Geometry: final body of the model. Coordinates: model frame, mm. Round coordinates to 2 decimals unless told otherwise and drop trailing zeros. Loops run counter-clockwise (first coordinate to the right, second up) from the corner with the lowest first, then second, coordinate; pieces in that order, holes last. Notation, with made-up numbers: (-36.75, 87) - (16.25, 87) arc R16 cw to (16.25, 93) - close; hole circle Ø11 at (87.5, -4). An arc over 180 degrees is marked (long way). Write item = value, one per line. Start each with the question number.
Item 1: Section B-B (y = 0.65). Count the separate pieces of the cut face and the enclosed holes in it, plus the area to 3 significant figures.
Item 2: First-contact query: pin 1 (8 mm diameter, centred on x = 13.5, z = 1.98, fed in from -Y); pin 2 (5.5 mm diameter, centred on x = -40.5, z = 1.98, fed in from +Y). Flat tips, straight axial feed; report the tip coordinate or a pass-through.
Item 3: Section A-A (x = -4.5). Return loops of the section in (y, z), plus the area to 3 significant figures.
Item 4: Draft query along X for faces 1 (the flat face through (-1, 0.794, -3)), 2 (the cylindrical face through (26.011, 0.391, -30.805)). Return one class per face: pulls with the +X half, pulls with the -X half, needs draft (parallel to the pull), parting line crosses it, or undercut.
from build123d import *

# Parameters (mm, degrees)
SKETCH1_W           = 108
SKETCH1_H           = 82
SKETCH1_R           = 1.625
SKETCH1_R_2         = 3.15
BOSS_EXTRUDE1_DEPTH = 0.79375


with BuildPart() as part:
    # Sketch1 → Boss-Extrude1 (new body)
    with BuildSketch(Plane(origin=(0, 0, 0), x_dir=(1, 0, 0), z_dir=(0, 1, 0))):
        with Locations((0, 2.515945223)):
            Rectangle(SKETCH1_W, SKETCH1_H)
        with Locations(Location((-45, 29.515945223, 0), (0, 0, 270))):
            Circle(SKETCH1_R, mode=Mode.SUBTRACT)
        with Locations(Location((-49.5, 25.015945223, 0), (0, 0, 270))):
            Circle(SKETCH1_R_2, mode=Mode.SUBTRACT)
        with Locations(Location((-27, 29.515945223, 0), (0, 0, 270))):
            Circle(SKETCH1_R, mode=Mode.SUBTRACT)
        with Locations(Location((-9, 29.515945223, 0), (0, 0, 270))):
            Circle(SKETCH1_R, mode=Mode.SUBTRACT)
        with Locations(Location((9, 29.515945223, 0), (0, 0, 270))):
            Circle(SKETCH1_R, mode=Mode.SUBTRACT)
        with Locations(Location((27, 29.515945223, 0), (0, 0, 270))):
            Circle(SKETCH1_R, mode=Mode.SUBTRACT)
        with Locations(Location((45, 29.515945223, 0), (0, 0, 270))):
            Circle(SKETCH1_R, mode=Mode.SUBTRACT)
        with Locations(Location((-27, 11.515945223, 0), (0, 0, 270))):
            Circle(SKETCH1_R, mode=Mode.SUBTRACT)
        with Locations(Location((-9, 11.515945223, 0), (0, 0, 270))):
            Circle(SKETCH1_R, mode=Mode.SUBTRACT)
        with Locations(Location((9, 11.515945223, 0), (0, 0, 270))):
            Circle(SKETCH1_R, mode=Mode.SUBTRACT)
        with Locations(Location((27, 11.515945223, 0), (0, 0, 270))):
            Circle(SKETCH1_R, mode=Mode.SUBTRACT)
        with Locations(Location((45, 11.515945223, 0), (0, 0, 270))):
            Circle(SKETCH1_R, mode=Mode.SUBTRACT)
        with Locations(Location((-27, -6.484054777, 0), (0, 0, 270))):
            Circle(SKETCH1_R, mode=Mode.SUBTRACT)
        with Locations(Location((-9, -6.484054777, 0), (0, 0, 270))):
            Circle(SKETCH1_R, mode=Mode.SUBTRACT)
        with Locations(Location((9, -6.484054777, 0), (0, 0, 270))):
            Circle(SKETCH1_R, mode=Mode.SUBTRACT)
        with Locations(Location((27, -6.484054777, 0), (0, 0, 270))):
            Circle(SKETCH1_R, mode=Mode.SUBTRACT)
        with Locations(Location((45, -6.484054777, 0), (0, 0, 270))):
            Circle(SKETCH1_R, mode=Mode.SUBTRACT)
        with Locations(Location((-27, -24.484054777, 0), (0, 0, 270))):
            Circle(SKETCH1_R, mode=Mode.SUBTRACT)
        with Locations(Location((-9, -24.484054777, 0), (0, 0, 270))):
            Circle(SKETCH1_R, mode=Mode.SUBTRACT)
        with Locations(Location((9, -24.484054777, 0), (0, 0, 270))):
            Circle(SKETCH1_R, mode=Mode.SUBTRACT)
        with Locations(Location((27, -24.484054777, 0), (0, 0, 270))):
            Circle(SKETCH1_R, mode=Mode.SUBTRACT)
        with Locations(Location((45, -24.484054777, 0), (0, 0, 270))):
            Circle(SKETCH1_R, mode=Mode.SUBTRACT)
        with Locations(Location((-45, 11.515945223, 0), (0, 0, 270))):
            Circle(SKETCH1_R, mode=Mode.SUBTRACT)
        with Locations(Location((-45, -6.484054777, 0), (0, 0, 270))):
            Circle(SKETCH1_R, mode=Mode.SUBTRACT)
        with Locations(Location((-45, -24.484054777, 0), (0, 0, 270))):
            Circle(SKETCH1_R, mode=Mode.SUBTRACT)
        with Locations(Location((-40.5, 25.015945223, 0), (0, 0, 270))):
            Circle(SKETCH1_R_2, mode=Mode.SUBTRACT)
        with Locations(Location((-31.5, 25.015945223, 0), (0, 0, 270))):
            Circle(SKETCH1_R_2, mode=Mode.SUBTRACT)
        with Locations(Location((-22.5, 25.015945223, 0), (0, 0, 270))):
            Circle(SKETCH1_R_2, mode=Mode.SUBTRACT)
        with Locations(Location((-13.5, 25.015945223, 0), (0, 0, 270))):
            Circle(SKETCH1_R_2, mode=Mode.SUBTRACT)
        with Locations(Location((-4.5, 25.015945223, 0), (0, 0, 270))):
            Circle(SKETCH1_R_2, mode=Mode.SUBTRACT)
        with Locations(Location((4.5, 25.015945223, 0), (0, 0, 270))):
            Circle(SKETCH1_R_2, mode=Mode.SUBTRACT)
        with Locations(Location((13.5, 25.015945223, 0), (0, 0, 270))):
            Circle(SKETCH1_R_2, mode=Mode.SUBTRACT)
        with Locations(Location((22.5, 25.015945223, 0), (0, 0, 270))):
            Circle(SKETCH1_R_2, mode=Mode.SUBTRACT)
        with Locations(Location((31.5, 25.015945223, 0), (0, 0, 270))):
            Circle(SKETCH1_R_2, mode=Mode.SUBTRACT)
        with Locations(Location((40.5, 25.015945223, 0), (0, 0, 270))):
            Circle(SKETCH1_R_2, mode=Mode.SUBTRACT)
        with Locations(Location((49.5, 25.015945223, 0), (0, 0, 270))):
            Circle(SKETCH1_R_2, mode=Mode.SUBTRACT)
        with Locations(Location((-40.5, 16.015945223, 0), (0, 0, 270))):
            Circle(SKETCH1_R_2, mode=Mode.SUBTRACT)
        with Locations(Location((-31.5, 16.015945223, 0), (0, 0, 270))):
            Circle(SKETCH1_R_2, mode=Mode.SUBTRACT)
        with Locations(Location((-22.5, 16.015945223, 0), (0, 0, 270))):
            Circle(SKETCH1_R_2, mode=Mode.SUBTRACT)
        with Locations(Location((-13.5, 16.015945223, 0), (0, 0, 270))):
            Circle(SKETCH1_R_2, mode=Mode.SUBTRACT)
        with Locations(Location((-4.5, 16.015945223, 0), (0, 0, 270))):
            Circle(SKETCH1_R_2, mode=Mode.SUBTRACT)
        with Locations(Location((4.5, 16.015945223, 0), (0, 0, 270))):
            Circle(SKETCH1_R_2, mode=Mode.SUBTRACT)
        with Locations(Location((13.5, 16.015945223, 0), (0, 0, 270))):
            Circle(SKETCH1_R_2, mode=Mode.SUBTRACT)
        with Locations(Location((22.5, 16.015945223, 0), (0, 0, 270))):
            Circle(SKETCH1_R_2, mode=Mode.SUBTRACT)
        with Locations(Location((31.5, 16.015945223, 0), (0, 0, 270))):
            Circle(SKETCH1_R_2, mode=Mode.SUBTRACT)
        with Locations(Location((40.5, 16.015945223, 0), (0, 0, 270))):
            Circle(SKETCH1_R_2, mode=Mode.SUBTRACT)
        with Locations(Location((49.5, 16.015945223, 0), (0, 0, 270))):
            Circle(SKETCH1_R_2, mode=Mode.SUBTRACT)
        with Locations(Location((-40.5, 7.015945223, 0), (0, 0, 270))):
            Circle(SKETCH1_R_2, mode=Mode.SUBTRACT)
        with Locations(Location((-31.5, 7.015945223, 0), (0, 0, 270))):
            Circle(SKETCH1_R_2, mode=Mode.SUBTRACT)
        with Locations(Location((-22.5, 7.015945223, 0), (0, 0, 270))):
            Circle(SKETCH1_R_2, mode=Mode.SUBTRACT)
        with Locations(Location((-13.5, 7.015945223, 0), (0, 0, 270))):
            Circle(SKETCH1_R_2, mode=Mode.SUBTRACT)
        with Locations(Location((-4.5, 7.015945223, 0), (0, 0, 270))):
            Circle(SKETCH1_R_2, mode=Mode.SUBTRACT)
        with Locations(Location((4.5, 7.015945223, 0), (0, 0, 270))):
            Circle(SKETCH1_R_2, mode=Mode.SUBTRACT)
        with Locations(Location((13.5, 7.015945223, 0), (0, 0, 270))):
            Circle(SKETCH1_R_2, mode=Mode.SUBTRACT)
        with Locations(Location((22.5, 7.015945223, 0), (0, 0, 270))):
            Circle(SKETCH1_R_2, mode=Mode.SUBTRACT)
        with Locations(Location((31.5, 7.015945223, 0), (0, 0, 270))):
            Circle(SKETCH1_R_2, mode=Mode.SUBTRACT)
        with Locations(Location((40.5, 7.015945223, 0), (0, 0, 270))):
            Circle(SKETCH1_R_2, mode=Mode.SUBTRACT)
        with Locations(Location((49.5, 7.015945223, 0), (0, 0, 270))):
            Circle(SKETCH1_R_2, mode=Mode.SUBTRACT)
        with Locations(Location((-40.5, -1.984054777, 0), (0, 0, 270))):
            Circle(SKETCH1_R_2, mode=Mode.SUBTRACT)
        with Locations(Location((-31.5, -1.984054777, 0), (0, 0, 270))):
            Circle(SKETCH1_R_2, mode=Mode.SUBTRACT)
        with Locations(Location((-22.5, -1.984054777, 0), (0, 0, 270))):
            Circle(SKETCH1_R_2, mode=Mode.SUBTRACT)
        with Locations(Location((-13.5, -1.984054777, 0), (0, 0, 270))):
            Circle(SKETCH1_R_2, mode=Mode.SUBTRACT)
        with Locations(Location((-4.5, -1.984054777, 0), (0, 0, 270))):
            Circle(SKETCH1_R_2, mode=Mode.SUBTRACT)
        with Locations(Location((4.5, -1.984054777, 0), (0, 0, 270))):
            Circle(SKETCH1_R_2, mode=Mode.SUBTRACT)
        with Locations(Location((13.5, -1.984054777, 0), (0, 0, 270))):
            Circle(SKETCH1_R_2, mode=Mode.SUBTRACT)
        with Locations(Location((22.5, -1.984054777, 0), (0, 0, 270))):
            Circle(SKETCH1_R_2, mode=Mode.SUBTRACT)
        with Locations(Location((31.5, -1.984054777, 0), (0, 0, 270))):
            Circle(SKETCH1_R_2, mode=Mode.SUBTRACT)
        with Locations(Location((40.5, -1.984054777, 0), (0, 0, 270))):
            Circle(SKETCH1_R_2, mode=Mode.SUBTRACT)
        with Locations(Location((49.5, -1.984054777, 0), (0, 0, 270))):
            Circle(SKETCH1_R_2, mode=Mode.SUBTRACT)
        with Locations(Location((-40.5, -10.984054777, 0), (0, 0, 270))):
            Circle(SKETCH1_R_2, mode=Mode.SUBTRACT)
        with Locations(Location((-31.5, -10.984054777, 0), (0, 0, 270))):
            Circle(SKETCH1_R_2, mode=Mode.SUBTRACT)
        with Locations(Location((-22.5, -10.984054777, 0), (0, 0, 270))):
            Circle(SKETCH1_R_2, mode=Mode.SUBTRACT)
        with Locations(Location((-13.5, -10.984054777, 0), (0, 0, 270))):
            Circle(SKETCH1_R_2, mode=Mode.SUBTRACT)
        with Locations(Location((-4.5, -10.984054777, 0), (0, 0, 270))):
            Circle(SKETCH1_R_2, mode=Mode.SUBTRACT)
        with Locations(Location((4.5, -10.984054777, 0), (0, 0, 270))):
            Circle(SKETCH1_R_2, mode=Mode.SUBTRACT)
        with Locations(Location((13.5, -10.984054777, 0), (0, 0, 270))):
            Circle(SKETCH1_R_2, mode=Mode.SUBTRACT)
        with Locations(Location((22.5, -10.984054777, 0), (0, 0, 270))):
            Circle(SKETCH1_R_2, mode=Mode.SUBTRACT)
        with Locations(Location((31.5, -10.984054777, 0), (0, 0, 270))):
            Circle(SKETCH1_R_2, mode=Mode.SUBTRACT)
        with Locations(Location((40.5, -10.984054777, 0), (0, 0, 270))):
            Circle(SKETCH1_R_2, mode=Mode.SUBTRACT)
        with Locations(Location((49.5, -10.984054777, 0), (0, 0, 270))):
            Circle(SKETCH1_R_2, mode=Mode.SUBTRACT)
        with Locations(Location((-40.5, -19.984054777, 0), (0, 0, 270))):
            Circle(SKETCH1_R_2, mode=Mode.SUBTRACT)
        with Locations(Location((-31.5, -19.984054777, 0), (0, 0, 270))):
            Circle(SKETCH1_R_2, mode=Mode.SUBTRACT)
        with Locations(Location((-22.5, -19.984054777, 0), (0, 0, 270))):
            Circle(SKETCH1_R_2, mode=Mode.SUBTRACT)
        with Locations(Location((-13.5, -19.984054777, 0), (0, 0, 270))):
            Circle(SKETCH1_R_2, mode=Mode.SUBTRACT)
        with Locations(Location((-4.5, -19.984054777, 0), (0, 0, 270))):
            Circle(SKETCH1_R_2, mode=Mode.SUBTRACT)
        with Locations(Location((4.5, -19.984054777, 0), (0, 0, 270))):
            Circle(SKETCH1_R_2, mode=Mode.SUBTRACT)
        with Locations(Location((13.5, -19.984054777, 0), (0, 0, 270))):
            Circle(SKETCH1_R_2, mode=Mode.SUBTRACT)
        with Locations(Location((22.5, -19.984054777, 0), (0, 0, 270))):
            Circle(SKETCH1_R_2, mode=Mode.SUBTRACT)
        with Locations(Location((31.5, -19.984054777, 0), (0, 0, 270))):
            Circle(SKETCH1_R_2, mode=Mode.SUBTRACT)
        with Locations(Location((40.5, -19.984054777, 0), (0, 0, 270))):
            Circle(SKETCH1_R_2, mode=Mode.SUBTRACT)
        with Locations(Location((49.5, -19.984054777, 0), (0, 0, 270))):
            Circle(SKETCH1_R_2, mode=Mode.SUBTRACT)
        with Locations(Location((-49.5, 16.015945223, 0), (0, 0, 270))):
            Circle(SKETCH1_R_2, mode=Mode.SUBTRACT)
        with Locations(Location((-49.5, 7.015945223, 0), (0, 0, 270))):
            Circle(SKETCH1_R_2, mode=Mode.SUBTRACT)
        with Locations(Location((-49.5, -1.984054777, 0), (0, 0, 270))):
            Circle(SKETCH1_R_2, mode=Mode.SUBTRACT)
        with Locations(Location((-49.5, -10.984054777, 0), (0, 0, 270))):
            Circle(SKETCH1_R_2, mode=Mode.SUBTRACT)
        with Locations(Location((-49.5, -19.984054777, 0), (0, 0, 270))):
            Circle(SKETCH1_R_2, mode=Mode.SUBTRACT)
    extrude(amount=BOSS_EXTRUDE1_DEPTH)


solid = part.part
Taken from the geometry:
q1.separate_pieces = 1
q1.enclosed_holes = 96
q1.area = 6,410 mm^2
q2.pin_1 = 0
q2.pin_2 = through
q3.outline = (0, -43.52) - (0.79, -43.52) - (0.79, -28.17) - (0, -28.17) - close; (0, -21.87) - (0.79, -21.87) - (0.79, -19.17) - (0, -19.17) - close; (0, -12.87) - (0.79, -12.87) - (0.79, -10.17) - (0, -10.17) - close; (0, -3.87) - (0.79, -3.87) - (0.79, -1.17) - (0, -1.17) - close; (0, 5.13) - (0.79, 5.13) - (0.79, 7.83) - (0, 7.83) - close; (0, 14.13) - (0.79, 14.13) - (0.79, 16.83) - (0, 16.83) - close; (0, 23.13) - (0.79, 23.13) - (0.79, 38.48) - (0, 38.48) - close
q3.area = 35.1 mm^2
q4.face_1 = needs draft
q4.face_2 = undercut
